Verification items for the finished model (mm, model axes). A direction names the side the tool comes from. Round coordinates to 2 decimals unless told otherwise and drop trailing zeros. Loops run counter-clockwise (first coordinate to the right, second up) from the corner with the lowest first, then second, coordinate; pieces in that order, holes last. Notation, with made-up numbers: (4.5, 9.25) - (46.5, 9.25) arc R20 ccw to (46.5, 38.25) - close; hole circle Ø9 at (22.25, -36.5). An arc over 180 degrees is marked (long way). Use a Markdown table: item, result. Add a question column.
```python
from build123d import *

# Parameters (mm, degrees)
SKETCH001_R      = 40
SKETCH001_R_2    = 12.5
EXTRUDE001_DEPTH = 1.6
SKETCH_R         = 18
SKETCH_R_2       = 1.55
SKETCH_R_3       = 1.6
SKETCH_R_4       = 3.5
SKETCH_R_5       = 1
EXTRUDE_DEPTH    = 5


with BuildPart() as extrude001:
    # Sketch001 (on Face7 of Extrude) → Extrude001 (new body)
    with BuildSketch(Plane.XY.offset(5)):
        Circle(SKETCH001_R)
        Circle(SKETCH001_R_2, mode=Mode.SUBTRACT)
    extrude(amount=-EXTRUDE001_DEPTH)


with BuildPart() as cut:
    # Sketch → Extrude (new body)
    with BuildSketch(Plane.XY):
        Circle(SKETCH_R)
        with Locations((0, 15)):
            Circle(SKETCH_R_2, mode=Mode.SUBTRACT)
        with Locations((-15, 0)):
            Circle(SKETCH_R_3, mode=Mode.SUBTRACT)
        with Locations((15, 0)):
            Circle(SKETCH_R_3, mode=Mode.SUBTRACT)
        with Locations((0, -15)):
            Circle(SKETCH_R_2, mode=Mode.SUBTRACT)
        Circle(SKETCH_R_4, mode=Mode.SUBTRACT)
        with Locations((0, 8)):
            Circle(SKETCH_R_5, mode=Mode.SUBTRACT)
        with Locations((6, 0)):
            Circle(SKETCH_R_5, mode=Mode.SUBTRACT)
        with Locations((0, -8)):
            Circle(SKETCH_R_5, mode=Mode.SUBTRACT)
        with Locations((-6, 0)):
            Circle(SKETCH_R_5, mode=Mode.SUBTRACT)
    extrude(amount=EXTRUDE_DEPTH)

    # Cut: cut Extrude001
    add(extrude001.part, mode=Mode.SUBTRACT)


solid = cut.part
```
Q1. Section check A-A on x = 0. Record the cut outline in (y, z).
Q2. Section check D-D on z = 2.9. State how many separate pieces and enclosed holes the cut face has, plus the area to 3 significant figures.
Q3. Go/stop test with flat-tipped pins: pin 1 Ø3 at (x, y) = (0.5, 8.5) entering from -Z; pin 2 Ø3 at (y, z) = (-5.5, 4) entering from -X; pin 3 Ø1.9 at (x, y) = (0, -15) entering from +Z; pin 4 Ø3 at (y, z) = (5, 4) entering from -X. Record where each tip stops, or that it passes through.
Q4. Release check for a two-part mould opening along Y. For faces 3 (the face through (13.4, 0.07, 1.68)), 4 (the face through (3, -3, 5)), 5 (the face through (11.923, 3.755, 4.211)) record: +Y half, -Y half, draft (parallel to the pull), parting line (faces both ways), or undercut.
Q5. Section check C-C on x = -6. Record the cut outline in (y, z).
Q6. Thickness scan on line 1 along Y through (x, z) = (0, 1.1); line 2 along X through (y, z) = (-14.5, 0.75); line 3 along Z through (x, y) = (15, 9). Record the ranges inside material, lowest first.
Q7. Set-up check for faces 1 (the face through (-4.1, 12.1, 3.4)), 2 (the face through (-0.202, -13.463, 1.676)): record each of +Z, -Z, +X, -X, +Y, -Y from which the full face is reachable in a straight line by a thin tool's end or side.
Q8. Section check B-B on y = 15. Record the cut outline in (x, z).
Determined:
| question | item | result |
|---|---|---|
| 1 | outline | (-18, 0) - (-16.55, 0) - (-16.55, 3.4) - (-18, 3.4) - close; (-13.45, 0) - (-9, 0) - (-9, 5) - (-12.5, 5) - (-12.5, 3.4) - (-13.45, 3.4) - close; (-7, 0) - (-3.5, 0) - (-3.5, 5) - (-7, 5) - close; (3.5, 0) - (7, 0) - (7, 5) - (3.5, 5) - close; (9, 0) - (13.45, 0) - (13.45, 3.4) - (12.5, 3.4) - (12.5, 5) - (9, 5) - close; (16.55, 0) - (18, 0) - (18, 3.4) - (16.55, 3.4) - close |
| 2 | separate pieces | 1 |
| 2 | enclosed holes | 9 |
| 2 | area | 936 mm² |
| 3 | pin 1 | stops at z = 0 |
| 3 | pin 2 | stops at x = -17.52 |
| 3 | pin 3 | passes through |
| 3 | pin 4 | stops at x = -17.63 |
| 4 | face 3 | undercut |
| 4 | face 4 | draft |
| 4 | face 5 | parting line |
| 5 | outline | (-16.97, 0) - (-1, 0) - (-1, 5) - (-10.97, 5) - (-10.97, 3.4) - (-16.97, 3.4) - close; (1, 0) - (16.97, 0) - (16.97, 3.4) - (10.97, 3.4) - (10.97, 5) - (1, 5) - close |
| 6 | line 1 | y = -18 to -16.55, -13.45 to -9, -7 to -3.5, 3.5 to 7, 9 to 13.45, 16.55 to 18 |
| 6 | line 2 | x = -10.67 to -1.47, 1.47 to 10.67 |
| 6 | line 3 | z = 0 to 3.4 |
| 7 | face 1 | +Z |
| 7 | face 2 | +Z, -Z |
| 8 | outline | (-9.95, 0) - (-1.55, 0) - (-1.55, 3.4) - (-9.95, 3.4) - close; (1.55, 0) - (9.95, 0) - (9.95, 3.4) - (1.55, 3.4) - close |
